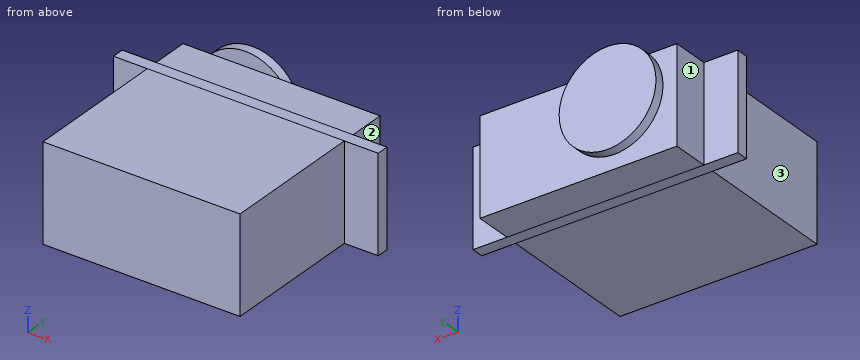
from build123d import *

# Parameters (mm, degrees)
SKETCH_1_W      = 40.7
SKETCH_1_H      = 19.9
EXTRUDE_1_DEPTH = 40
SKETCH_2_R      = 3
EXTRUDE_2_DEPTH = 6
EXTRUDE_START   = -7.7
SKETCH_3_W      = 54.7
SKETCH_3_H      = 19.901230414
EXTRUDE_3_DEPTH = 2.5
SKETCH_4_R      = 10
EXTRUDE_4_DEPTH = 2


with BuildPart() as part:
    # 스케치1 → 보스-돌출1 (new body)
    with BuildSketch(Plane(origin=(0, 0, 0), x_dir=(1, 0, 0), z_dir=(0, 1, 0))):
        Rectangle(SKETCH_1_W, SKETCH_1_H)
    extrude(amount=EXTRUDE_1_DEPTH)

    # 스케치2 → 보스-돌출2 (add)
    with BuildSketch(Plane(origin=(0, 40, 0), x_dir=(1, 0, 0), z_dir=(0, 1, 0))):
        with Locations(Location((-10.35, 0, 0), (0, 0, 270))):
            Circle(SKETCH_2_R)
    extrude(amount=EXTRUDE_2_DEPTH)

    # 스케치3 → 보스-돌출3 (add)
    with BuildSketch(Plane(origin=(0, 40, 0), x_dir=(1, 0, 0), z_dir=(0, 1, 0)).offset(EXTRUDE_START)):
        Rectangle(SKETCH_3_W, SKETCH_3_H)
    extrude(amount=-EXTRUDE_3_DEPTH)

    # 스케치4 → 보스-돌출4 (add)
    with BuildSketch(Plane(origin=(0, 46, 0), x_dir=(1, 0, 0), z_dir=(0, 1, 0))):
        with Locations(Location((-10.35, 0, 0), (0, 0, 270))):
            Circle(SKETCH_4_R)
    extrude(amount=-EXTRUDE_4_DEPTH)


solid = part.part
Can you work these out from the model? Positions are in its coordinate system, mm. Face numbers are marked on the shaded views. A direction names the side the tool comes from. Give positions to 0.01 mm unless a question says otherwise; leave off trailing zeros. Loops run counter-clockwise (first coordinate to the right, second up) from the corner with the lowest first, then second, coordinate; pieces in that order, holes last. Notation, with made-up numbers: (-31.5, -15.5) -> (-6.5, -15.5) arc R25 ccw to (-6.5, 16.5) -> close; hole circle Ø1 at (61.5, -1). An arc over 180 degrees is marked (long way). Write item = value, one per line.
1) Will these pins go through, and if not, where does the flat tip stop? pin 1 (4 mm diameter, centred on x = 4.5, y = 23.5, fed in from +Z); pin 2 (10 mm diameter, centred on x = -2, y = 37, fed in from -Z); pin 3 (10 mm diameter, centred on y = 20, z = -5, fed in from +X).
Check result:
pin_1 = 9.95
pin_2 = -9.95
pin_3 = 20.35
2) Suppose I cut it at C-C on z = 0. Write out the boundary of the cut face in (x, y).
Check result:
outline = (-27.35, 29.8) -> (-20.35, 29.8) -> (-20.35, 0) -> (20.35, 0) -> (20.35, 29.8) -> (27.35, 29.8) -> (27.35, 32.3) -> (20.35, 32.3) -> (20.35, 40) -> (-7.35, 40) -> (-7.35, 44) -> (-0.35, 44) -> (-0.35, 46) -> (-20.35, 46) -> (-20.35, 44) -> (-13.35, 44) -> (-13.35, 40) -> (-20.35, 40) -> (-20.35, 32.3) -> (-27.35, 32.3) -> close
3) For the marked faces 1, 2 and 3, which set-ups out of +Z, -Z, +X, -X, +Y, -Y let a thin tool reach every point of the face, with its end or its side?
Check result:
face_1 = +Z, -Z, -X, +Y
face_2 = +Z, -Z, +X, +Y
face_3 = +Z, -Z, -X, -Y
4) Suppose I cut it at D-D on x = -22. Write out the boundary of the cut face in (y, z), then the cut area to 3 significant figures.
Check result:
outline = (29.8, -9.95) -> (32.3, -9.95) -> (32.3, 9.95) -> (29.8, 9.95) -> close
area = 49.8 mm2
5) I need wall thicknesses on L1, parallel to Y at x = -7, z = -8.5; L2, parallel to Z at x = 17, y = 14; L3, parallel to X at y = 34, z = 4.5. Which ranges of each line are inside material? Lowest first, please. Write a range as from..to.
Check result:
L1 = 0..40, 44..46
L2 = -9.95..9.95
L3 = -20.35..20.35
6) Suppose I cut it at A-A on z = -6. Write out the boundary of the cut face in (x, y).
Check result:
outline = (-27.35, 29.8) -> (-20.35, 29.8) -> (-20.35, 0) -> (20.35, 0) -> (20.35, 29.8) -> (27.35, 29.8) -> (27.35, 32.3) -> (20.35, 32.3) -> (20.35, 40) -> (-20.35, 40) -> (-20.35, 32.3) -> (-27.35, 32.3) -> close; (-18.35, 44) -> (-2.35, 44) -> (-2.35, 46) -> (-18.35, 46) -> close
